```python
from build123d import *

# Parameters (mm, degrees)
BOSS_EXTRU_1_DEPTH      = 6
ESQUISSE14_R            = 1.5
ENL_V_MAT_EXTRU_1_DEPTH = 8


with BuildPart() as part:
    # Esquisse13 → Boss.-Extru.1 (new body)
    with BuildSketch(Plane.XY):
        Polygon((0.044605576, 12.611770032), (-10.948101074, -6.248487138), (10.881714082, -6.338321768), align=None)
    extrude(amount=BOSS_EXTRU_1_DEPTH)

    # Esquisse14 → Enlèv. mat.-Extru.1 (cut)
    with BuildSketch(Plane.XY.offset(6)):
        with Locations((0.025841827, 7.991160973)):
            Circle(ESQUISSE14_R)
        with Locations((6.891022326, -4.010372012)):
            Circle(ESQUISSE14_R)
        with Locations((-6.937774801, -3.955049343)):
            Circle(ESQUISSE14_R)
    extrude(amount=-ENL_V_MAT_EXTRU_1_DEPTH, mode=Mode.SUBTRACT)


solid = part.part
```
Check sheet for the modelled part. Datum: model origin and axes. Units: mm. Round coordinates to 2 decimals unless told otherwise and drop trailing zeros. Loops run counter-clockwise (first coordinate to the right, second up) from the corner with the lowest first, then second, coordinate; pieces in that order, holes last. Notation, with made-up numbers: M 68,-29 L 89,-29 A17 ccw 89,-5 Z; hole C 19,16.5 d10. An arc over 180 degrees is marked long. Answer as a JSON object with one key per item and string values.
1. Mould release check, pull along Y, two halves, no side actions. Record for faces 1 (the cylindrical face through (8.32, -3.56, 3.04)), 2 (the flat face through (-5.375, 3.314, 2.958)), 3 (the flat face through (0, 1, 0)), 4 (the cylindrical face through (-0.17, 9.48, 3.04)): pulls with the +Y half, pulls with the -Y half, needs draft (parallel to the pull), parting line crosses it, or undercut.
Reply:
{"face 1": "undercut", "face 2": "pulls with the +Y half", "face 3": "needs draft", "face 4": "undercut"}
2. Section check B-B (y = -3.5). Record the boundary of the cut face in (x, z), plus the area to 3 significant figures.
Reply:
{"outline": "M -9.35,0 L -8.37,0 L -8.37,6 L -9.35,6 Z; M -5.51,0 L 5.48,0 L 5.48,6 L -5.51,6 Z; M 8.3,0 L 9.26,0 L 9.26,6 L 8.3,6 Z", "area": "77.6 mm²"}
3. Section check D-D (z = 5.3). Record the boundary of the cut face in (x, y), plus the area to 3 significant figures.
Reply:
{"outline": "M -10.95,-6.25 L 10.88,-6.34 L 0.04,12.61 Z; hole C -6.94,-3.96 d3; hole C 0.03,7.99 d3; hole C 6.89,-4.01 d3", "area": "185 mm²"}
4. Section check A-A (x = -7). Record the boundary of the cut face in (y, z), plus the area to 3 significant figures.
Reply:
{"outline": "M -6.26,0 L -5.45,0 L -5.45,6 L -6.26,6 Z; M -2.46,0 L 0.53,0 L 0.53,6 L -2.46,6 Z", "area": "22.8 mm²"}
5. Gauge pin test, flat ends, axial feed: P1, Ø3, axis at x = 6, z = 5, coming from the +Y side; P2, Ø2.5, axis at x = -6.94, y = -3.96, coming from the +Z side; P3, Ø1.5, axis at y = 8.5, z = 3.5, coming from the -X side; P4, Ø3, axis at x = 4.5, z = 0.5, coming from the -Y side. Record the tip position at first contact, or that the pin passes through.
Reply:
{"P1": "stops at y = 4.82", "P2": "passes through", "P3": "stops at x = -2.79", "P4": "stops at y = -6.32"}
6. Section check C-C (y = 6.75). Record the boundary of the cut face in (x, z), plus the area to 3 significant figures.
Reply:
{"outline": "M -3.37,0 L -0.82,0 L -0.82,6 L -3.37,6 Z; M 0.87,0 L 3.4,0 L 3.4,6 L 0.87,6 Z", "area": "30.5 mm²"}
7. Scan lines: line 1 (X direction, y = -3, z = 5.75); line 2 (X direction, y = -2.75, z = 0.35); line 3 (X direction, y = 7, z = 4.05). Record each from-to range of solid material in increasing order.
Reply:
{"line 1": "x = -9.05 to -8.09, -5.78 to 5.78, 8 to 8.97", "line 2": "x = -8.91 to -7.83, -6.04 to 6.08, 7.7 to 8.83", "line 3": "x = -3.23 to -1.1, 1.15 to 3.25"}
